Check sheet for the drawn part. Datum: minimum x, y, z corner. Units: mm. Round coordinates to 2 decimals unless told otherwise and drop trailing zeros. Order: outer loops, then holes, each group sorted by start corner. A loop starts at its lowest first (then second) coordinate and runs counter-clockwise, first axis right, second up. Notation, with made-up numbers: M 31,58 L 63,58 A35 ccw 63,91 Z; hole C -35.5,87 d6. An arc over 180 degrees is marked long. Use one line per item in the form item = value. Start each with the question number.
Item 1: Cross-section at A-A on x = 96. Count the separate pieces of the cut face and the enclosed holes in it, then the cut area to 3 significant figures.
Item 2: Thickness scan on probe 1 along Y at (x, z) = (142.5, 45); probe 2 along Z at (x, y) = (149, 42.5); probe 3 along Z at (x, y) = (165.5, 70.5). Record the ranges inside material, lowest first. Write a range as [from, to].
Item 3: Go/stop test with flat-tipped pins: pin 1 Ø20.5 at (x, z) = (73.5, 41.5) entering from +Y; pin 2 Ø20.5 at (x, y) = (81.5, 104) entering from +Z; pin 3 Ø8 at (y, z) = (70.5, 31.5) entering from +X. Record where each tip stops, or that it passes through.
Item 4: Cross-section at C-C on y = 98. Enter the section's corners in (x, z), then the cut area to 3 significant figures.
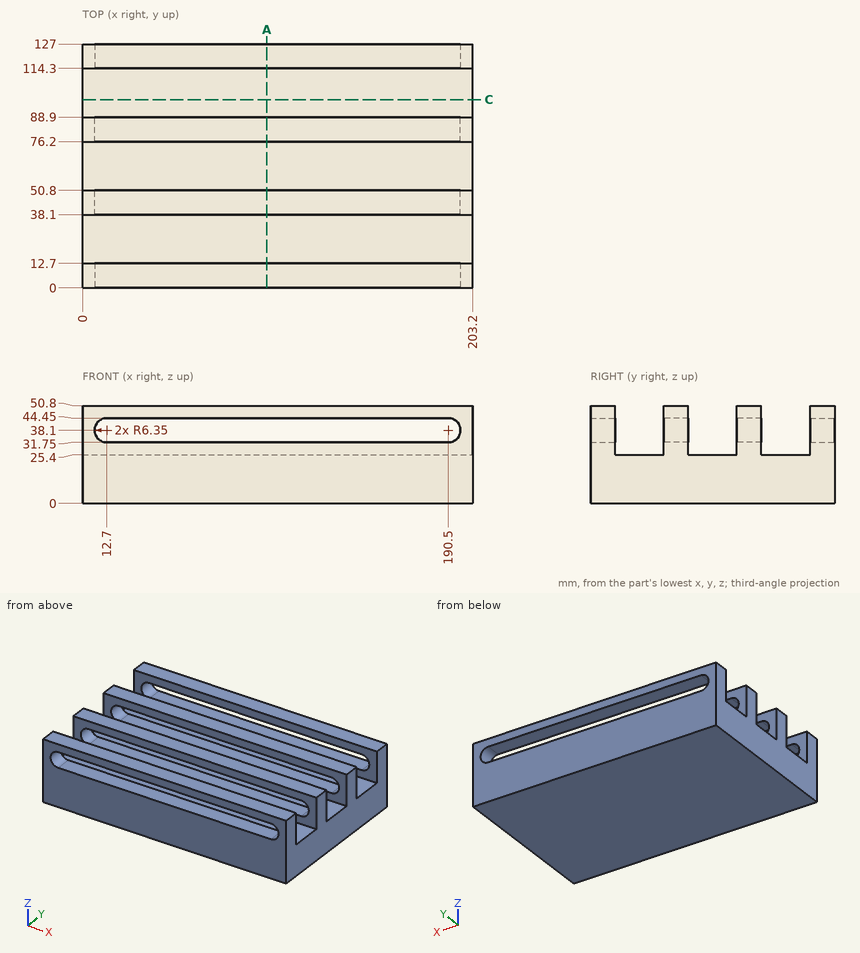
Output values:
q1.separate_pieces = 5
q1.enclosed_holes = 0
q1.area = 3,870 mm2
q2.probe_1 = [0, 12.7], [38.1, 50.8], [76.2, 88.9], [114.3, 127]
q2.probe_2 = [0, 31.75], [44.45, 50.8]
q2.probe_3 = [0, 25.4]
q3.pin_1 = 127
q3.pin_2 = 25.4
q3.pin_3 = through
q4.outline = M 0,0 L 203.2,0 L 203.2,25.4 L 0,25.4 Z
q4.area = 5,160 mm2
